from build123d import *

# Parameters (mm, degrees)
HOLE_WIZARD_5_2_5_2_1_D           = 5.2
HOLE_WIZARD_5_2_5_2_1_CSINK_D     = 5.25
HOLE_WIZARD_5_2_5_2_1_CSINK_ANGLE = 90
SKETCH_4_W                        = 4
SKETCH_4_H                        = 4.736079205
CUT_EXTRUDE_1_DEPTH               = 35


with BuildPart() as part:
    # 草图1 → 旋转1 (revolve)
    with BuildSketch(Plane.XY, mode=Mode.PRIVATE) as revolve_1_sk:
        Polygon((0, 6), (0, 15), (20.4, 15), (20.4, 22.72), (26.4, 22.72), (26.4, 6), align=None)
    revolve(revolve_1_sk.sketch.rotate(Axis((0, 0, 0), (1, 0, 0)), 90), axis=Axis((0, 0, 0), (1, 0, 0)))

    # Ø5.2 (5.2) 直径孔1 (through all)
    with Locations(Plane.ZY.offset(-20.4)):
        with Locations((0, 18.8), (16.281277591, -9.4), (-16.281277591, -9.4), (0, -18.8), (-16.281277591, 9.4), (16.281277591, 9.4)):
            CounterSinkHole(HOLE_WIZARD_5_2_5_2_1_D / 2, HOLE_WIZARD_5_2_5_2_1_CSINK_D / 2, counter_sink_angle=HOLE_WIZARD_5_2_5_2_1_CSINK_ANGLE)

    # 草图4 → 切除-拉伸1 (cut)
    with BuildSketch(Plane.ZY):
        with Locations((0, 5.231960397)):
            Rectangle(SKETCH_4_W, SKETCH_4_H)
    extrude(amount=-CUT_EXTRUDE_1_DEPTH, mode=Mode.SUBTRACT)


solid = part.part
Verification items for the finished model (mm, model axes). A direction names the side the tool comes from. Round coordinates to 2 decimals unless told otherwise and drop trailing zeros. Loops run counter-clockwise (first coordinate to the right, second up) from the corner with the lowest first, then second, coordinate; pieces in that order, holes last. Notation, with made-up numbers: (55.5, -34.75) - (104.5, -34.75) arc R23 ccw to (104.5, -13.75) - close; hole circle Ø11 at (-10.75, -9.75). An arc over 180 degrees is marked (long way). Write item = value, one per line.
Q1. Sectioned sample at C-C on y = -4. Record the boundary of the cut face in (x, z).
Here are the results:
outline = (0, -14.46) - (20.4, -14.46) - (20.4, -22.37) - (26.4, -22.37) - (26.4, -4.47) - (0, -4.47) - close; (0, 4.47) - (26.4, 4.47) - (26.4, 22.37) - (20.4, 22.37) - (20.4, 14.46) - (0, 14.46) - close
Q2. Mould release check, pull along Y, two halves, no side actions. Record for faces 4 (the flat face through (0, -0.2, -6.5)), 5 (the cylindrical face through (23.45, -8.62, 13.8)), 6 (the cylindrical face through (23.442, -22.527, -2.958)): +Y half, -Y half, draft (parallel to the pull), parting line (faces both ways), or undercut.
Here are the results:
face_4 = draft
face_5 = undercut
face_6 = parting line
Q3. Sectioned sample at A-A on x = 23.5. Record the boundary of the cut face in (y, z).
Here are the results:
outline = circle Ø45.44 at (0, 0); hole circle Ø5.2 at (-18.8, 0); hole circle Ø5.2 at (-9.4, -16.28); hole circle Ø5.2 at (-9.4, 16.28); hole (5.66, -2) - (7.6, -2) - (7.6, 2) - (5.66, 2) arc R6 ccw (long way) to start; hole circle Ø5.2 at (9.4, -16.28); hole circle Ø5.2 at (9.4, 16.28); hole circle Ø5.2 at (18.8, 0)
Q4. Tool access check on faces 1 (the flat face through (20.4, 5, -15)), 2 (the flat face through (26.4, 5, 5)), 3 (the flat face through (13, 7, -2)). Record the directions out of +Z, -Z, +X, -X, +Y, -Y that give a thin tool (end or side, any length) a straight path to the whole face; none if there is none.
Here are the results:
face_1 = -X
face_2 = +Z, -Z, +X, +Y, -Y
face_3 = +X, -X
Q5. Sectioned sample at B-B on z = 0. Record the boundary of the cut face in (x, y) (3 decimals), plus the area to 3 significant figures.
Here are the results:
outline = (0, -15) - (20.4, -15) - (20.4, -16.175) - (20.425, -16.2) - (26.4, -16.2) - (26.4, -6) - (0, -6) - close; (0, 7.6) - (26.4, 7.6) - (26.4, 16.2) - (20.425, 16.2) - (20.4, 16.175) - (20.4, 15) - (0, 15) - close; (20.4, -22.72) - (26.4, -22.72) - (26.4, -21.4) - (20.425, -21.4) - (20.4, -21.425) - close; (20.4, 21.425) - (20.425, 21.4) - (26.4, 21.4) - (26.4, 22.72) - (20.4, 22.72) - close
area = 463 mm^2
Q6. Depth check by flat-ended pin: pin 1 (4 mm diameter, centred on x = 20.5, y = 10, fed in from -Z); pin 2 (4 mm diameter, centred on x = 22.5, y = -13, fed in from +Z); pin 3 (8 mm diameter, centred on x = 18, z = 3, fed in from -Y). Enter the tip coordinate at first touch or a pass-through.
Here are the results:
pin_1 = -21.26
pin_2 = 19.88
pin_3 = -22.72
Q7. Material ranges on L1, parallel to Y at x = 24.75, z = 0; L2, parallel to X at y = 15, z = -13; L3, parallel to Z at x = 23.65, y = -9.4, recorded low to high.
Here are the results:
L1 = -22.72 to -21.4, -16.2 to -6, 7.6 to 16.2, 21.4 to 22.72
L2 = 20.4 to 26.4
L3 = -20.68 to -18.88, -13.68 to 13.68, 18.88 to 20.68
Q8. Sectioned sample at D-D on x = 4.5. Record the boundary of the cut face in (y, z).
Here are the results:
outline = circle Ø30 at (0, 0); hole (5.66, -2) - (7.6, -2) - (7.6, 2) - (5.66, 2) arc R6 ccw (long way) to start
